Build history of the part. All positions in model axes, mm. Give positions to 0.01 mm unless a question says otherwise; leave off trailing zeros. Write each loop counter-clockwise with the first axis right and the second up, starting at its lowest first coordinate (ties: lowest second). Pieces come first, ordered by that corner, then holes. Notation, with made-up numbers: (56, -20.5) -> (74, -20.5) arc R23 ccw to (74, -2.5) -> close; hole circle Ø10 at (-29, 81). An arc over 180 degrees is marked (long way). Write item = value, one per line. Start each with the question number.
Q1. Saw through at C-C, the plane z = 6. List the corners of the cut face in (x, y).
Q2. Drop flat-ended pins along their axis: P1, Ø5, axis at y = 55.5, z = 7.5, coming from the +X side; P2, Ø5, axis at y = -17, z = 4, coming from the -X side; P3, Ø8, axis at x = 0, y = 79, coming from the -Z side. Give the stop position or say it passes through.
Q3. Saw through at A-A, the plane x = 0. List the corners of the cut face in (y, z), then the cut area to 3 significant figures.
Q4. Wall check: line 1 (Y direction, x = 0, z = 3.5); line 2 (Y direction, x = -36.5, z = 7.5); line 3 (Y direction, x = -79, z = 7). Give the ranges that are in metal, low to high.
Q5. Mould opens along X. For faces 1 (the face through (-45.3, 58.1, 0)), 2 (the face through (1.15, 76.78, 5.31)), 3 (the face through (-68.643, -52.634, 4.19)), 4 (the face through (76.5, 0.1, 5.3)) say: pulls with the +X half, pulls with the -X half, needs draft (parallel to the pull), parting line crosses it, or undercut.
Q6. Saw through at B-B, the plane y = 17.5. List the corners of the cut face in (x, z).
Q7. Saw through at D-D, the plane x = -69. List the corners of the cut face in (y, z).
from build123d import *

# Parameters (mm, degrees)
SKETCH_1_R                   = 86.5
SKETCH_1_R_2                 = 73.5
SKETCH_1_R_3                 = 2.5
EXTRUDE_1_DEPTH              = 8.5
HOLE_WIZARD_M4_1_D           = 4.8
HOLE_WIZARD_M4_1_CSINK_D     = 9.4
HOLE_WIZARD_M4_1_CSINK_ANGLE = 90


with BuildPart() as part:
    # ｽｹｯﾁ1 → ﾎﾞｽ - 押し出し1 (new body)
    with BuildSketch(Plane.XY):
        Circle(SKETCH_1_R)
        Circle(SKETCH_1_R_2, mode=Mode.SUBTRACT)
        with Locations((0, 79)):
            Circle(SKETCH_1_R_3, mode=Mode.SUBTRACT)
        with Locations((79, 0)):
            Circle(SKETCH_1_R_3, mode=Mode.SUBTRACT)
        with Locations((0, -79)):
            Circle(SKETCH_1_R_3, mode=Mode.SUBTRACT)
        with Locations((-79, 0)):
            Circle(SKETCH_1_R_3, mode=Mode.SUBTRACT)
    extrude(amount=EXTRUDE_1_DEPTH)

    # M4 丸皿ねじ用皿穴1 (through all)
    with Locations(Plane(origin=(0, 0, 0), x_dir=(-1, 0, 0), z_dir=(0, 0, -1))):
        with Locations((-79, 0), (79, 0), (0, 79), (0, -79)):
            CounterSinkHole(HOLE_WIZARD_M4_1_D / 2, HOLE_WIZARD_M4_1_CSINK_D / 2, counter_sink_angle=HOLE_WIZARD_M4_1_CSINK_ANGLE)


solid = part.part
Report:
q1.outline = circle Ø173 at (0, 0); hole circle Ø5 at (-79, 0); hole circle Ø147 at (0, 0); hole circle Ø5 at (0, -79); hole circle Ø5 at (0, 79); hole circle Ø5 at (79, 0)
q2.P1 = 68.36
q2.P2 = -85.28
q2.P3 = 0.7
q3.outline = (-86.5, 0) -> (-83.7, 0) -> (-81.5, 2.2) -> (-81.5, 8.5) -> (-86.5, 8.5) -> close; (-76.5, 2.2) -> (-74.3, 0) -> (-73.5, 0) -> (-73.5, 8.5) -> (-76.5, 8.5) -> close; (73.5, 0) -> (74.3, 0) -> (76.5, 2.2) -> (76.5, 8.5) -> (73.5, 8.5) -> close; (81.5, 2.2) -> (83.7, 0) -> (86.5, 0) -> (86.5, 8.5) -> (81.5, 8.5) -> close
q3.area = 126 mm2
q4.line_1 = -86.5 to -81.5, -76.5 to -73.5, 73.5 to 76.5, 81.5 to 86.5
q4.line_2 = -78.42 to -63.8, 63.8 to 78.42
q4.line_3 = -35.23 to -2.5, 2.5 to 35.23
q5.face_1 = needs draft
q5.face_2 = undercut
q5.face_3 = parting line crosses it
q5.face_4 = undercut
q6.outline = (-84.71, 0) -> (-71.39, 0) -> (-71.39, 8.5) -> (-84.71, 8.5) -> close; (71.39, 0) -> (84.71, 0) -> (84.71, 8.5) -> (71.39, 8.5) -> close
q7.outline = (-52.17, 0) -> (-25.32, 0) -> (-25.32, 8.5) -> (-52.17, 8.5) -> close; (25.32, 0) -> (52.17, 0) -> (52.17, 8.5) -> (25.32, 8.5) -> close
